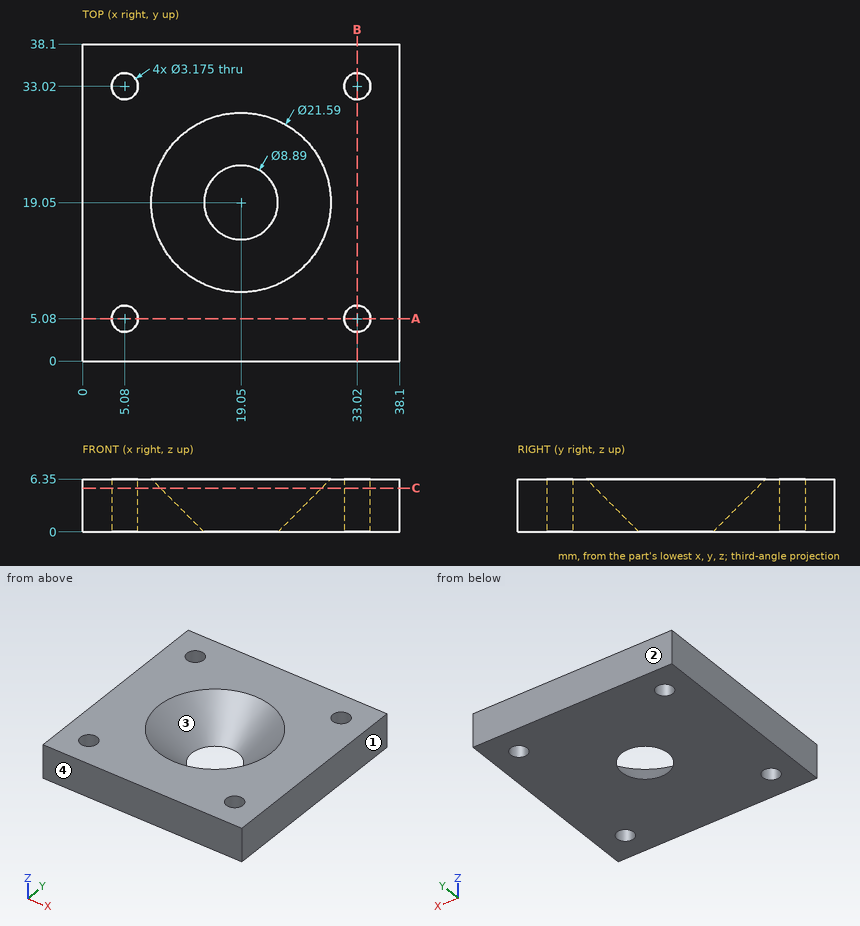
Part print with two shaded views. Sizes in mm from the minimum x, y, z corner. Round coordinates to 2 decimals unless told otherwise and drop trailing zeros. Order: outer loops, then holes, each group sorted by start corner. A loop starts at its lowest first (then second) coordinate and runs counter-clockwise, first axis right, second up. Notation, with made-up numbers: (41.25, 50.5) - (85.25, 50.5) arc R17 ccw to (85.25, 69.5) - close; hole circle Ø5 at (69, 54.5). An arc over 180 degrees is marked (long way). Return JSON: item names as keys, results as strings.
(1) Cut at A-A (y = 5.08). Give the cut face in (x, z), then the cut area to 3 significant figures.
Answer key:
{"outline": "(0, 0) - (3.49, 0) - (3.49, 6.35) - (0, 6.35) - close; (6.67, 0) - (31.43, 0) - (31.43, 6.35) - (6.67, 6.35) - close; (34.61, 0) - (38.1, 0) - (38.1, 6.35) - (34.61, 6.35) - close", "area": "202 mm^2"}
(2) Cut at C-C (z = 5.25). State how many separate pieces and enclosed holes the cut face has, then the cut area to 3 significant figures.
Answer key:
{"separate pieces": "1", "enclosed holes": "5", "area": "1,120 mm^2"}
(3) Pull direction Y, two halves, no side cores. Call the marked faces 1, 2, 3 and 4: +Y half, -Y half, draft (parallel to the pull), parting line (faces both ways), or undercut.
Answer key:
{"face 1": "draft", "face 2": "+Y half", "face 3": "undercut", "face 4": "-Y half"}
(4) Wall check: probe 1 along Y at (x, z) = (5.08, 2.5); probe 2 along X at (y, z) = (4, 4). Give the ranges that are in metal, low to high. Write a range as from..to.
Answer key:
{"probe 1": "y = 0..3.49, 6.67..31.43, 34.61..38.1", "probe 2": "x = 0..3.92, 6.24..31.86, 34.18..38.1"}
